Work out the finished part from the listing and answer in its coordinate system (mm). Give positions to 0.01 mm unless a question says otherwise; leave off trailing zeros. Write each loop counter-clockwise with the first axis right and the second up, starting at its lowest first coordinate (ties: lowest second). Pieces come first, ordered by that corner, then holes. Notation, with made-up numbers: (-35, 54) - (-21, 54) arc R19 cw to (-21, 91) - close; hole circle Ø8 at (0, -25.5). An arc over 180 degrees is marked (long way). Write item = value, one per line.
from build123d import *

# Parameters (mm, degrees)
F0_R     = 4.149094
F1_DEPTH = 2.54
F3_DEPTH = 25.4
F4_DEPTH = 25.4
F6_DEPTH = 25.4


with BuildPart() as f1:
    # F0 (on Front) → F1 (new body)
    with BuildSketch(Plane.XZ):
        with BuildLine():
            Line((-9.525, 6.705717), (-9.525, -4.406783))
            Line((-9.525, -4.406783), (0, -4.406783))
            Line((0, -4.406783), (0, -4.615923))
            ThreePointArc((0, -4.615923), (2.094218, 0.756224), (7.271803, 3.293612))
            Line((7.271803, 3.293612), (66.675, 8.293217))
            Line((66.675, 8.293217), (66.675, 14.643217))
            Line((66.675, 14.643217), (-1.5875, 14.643217))
            ThreePointArc((-1.5875, 14.643217), (-7.20016, 12.318377), (-9.525, 6.705717))
        make_face()
        with Locations((-3.333452, 8.143553)):
            Circle(F0_R, mode=Mode.SUBTRACT)
    extrude(amount=F1_DEPTH)

    # F2 (on face) → F3 (cut)
    with BuildSketch(Plane(origin=(-9.525, 0, 0), x_dir=(0, -1, 0), z_dir=(-1, 0, 0))):
        Polygon((2.54, -4.406783), (2.54, 3.190069), (0.604368, -4.406783), align=None)
    extrude(amount=-F3_DEPTH, mode=Mode.SUBTRACT)

    # F1_face (on face) → F4 (cut)
    with BuildSketch(Plane(origin=(-9.525, -1.27, 1.149467), x_dir=(0, -1, 0), z_dir=(-1, 0, 0))):
        Polygon((-0.665632, -5.55625), (-1.27, -5.55625), (-1.27, -5.76539), (1.27, -5.76539), (1.27, -5.55625), align=None)
    extrude(amount=-F4_DEPTH, mode=Mode.SUBTRACT)

    # F5 (on face) → F6 (cut)
    with BuildSketch(Plane.XY.offset(14.643217)):
        Polygon((66.675, 0), (50.660294, 0), (66.675, -1.27), align=None)
        Polygon((66.675, -1.524), (50.660294, -2.54), (66.675, -2.54), align=None)
    extrude(amount=-F6_DEPTH, mode=Mode.SUBTRACT)


solid = f1.part
1. Straight lines are drawn through the part: line 1 (Z direction, x = 43, y = -0.55); line 2 (X direction, y = -0.2, z = 1.25) (3 decimals); line 3 (Z direction, x = 21, y = -1.55). For each, find the intervals that lie inside material, in ascending order.
Solution:
line_1 = 6.3 to 14.64
line_2 = -9.525 to 2.59
line_3 = 4.45 to 14.64
2. Find section A-A, the plane z = 9.5. Give the vertices of the cut face in (x, y) (3 decimals).
Solution:
outline = (-9.017, -2.54) - (-7.255, -2.54) - (-7.255, 0) - (-9.017, 0) - close; (0.588, -2.54) - (50.66, -2.54) - (66.675, -1.524) - (66.675, -1.27) - (50.66, 0) - (0.588, 0) - close
3. Find section B-B, the plane y = -1.95. Give the vertices of the cut face in (x, z) (1 decimal).
Solution:
outline = (-9.5, 0.9) - (2.2, 0.9) arc R7.9 cw to (7.3, 3.3) - (60, 7.7) - (60, 14.6) - (-1.6, 14.6) arc R7.9 ccw to (-9.5, 6.7) - close; hole circle Ø8.3 at (-3.3, 8.1)
4. For a pull along X with two mould halves and no side action, classify faces 1 (the cylindrical face through (-6.626, -1.252, 5.619)), 2 (the cylindrical face through (-7.14, -1.25, 12.38)), 3 (the flat face through (58.78, -2.025, 10.848)) as pulls with the +X half, pulls with the -X half, needs draft (parallel to the pull), parting line crosses it, or undercut.
Solution:
face_1 = undercut
face_2 = pulls with the -X half
face_3 = pulls with the +X half
5. Find section C-C, the plane z = 5.5. Give the vertices of the cut face in (x, y) (3 decimals), then the cut area to 3 significant figures.
Solution:
outline = (-9.525, -2.54) - (-6.531, -2.54) - (-6.531, 0) - (-9.525, 0) - close; (-0.136, -2.54) - (33.487, -2.54) - (33.487, 0) - (-0.136, 0) - close
area = 93.0 mm^2
6. Given pin 1 (4 mm diameter, centred on x = 22.5, z = 2.5, fed in from -Y), flat-ended and moving along its own axis, determine where the tip first touches the part or whether it passes through.
Solution:
pin_1 = through
7. Find section D-D, the plane x = 33. Give the vertices of the cut face in (y, z), then the cut area to 3 significant figures.
Solution:
outline = (-2.54, 5.46) - (0, 5.46) - (0, 14.64) - (-2.54, 14.64) - close
area = 23.3 mm^2
